from build123d import *

# Parameters (mm, degrees)
SKETCH1_W           = 13
SKETCH1_H           = 16.2
BOSS_EXTRUDE1_DEPTH = 12.5
SKETCH2_W           = 2
SKETCH2_H           = 16.2
BOSS_EXTRUDE5_DEPTH = 6.5
SKETCH7_R           = 2.9
BOSS_EXTRUDE6_DEPTH = 2.5
SKETCH8_R           = 1.9
BOSS_EXTRUDE7_DEPTH = 8
SKETCH9_W           = 5
SKETCH9_H           = 16.2
BOSS_EXTRUDE8_DEPTH = 4
SKETCH10_W          = 0.8
SKETCH10_H          = 9.3
CUT_EXTRUDE3_DEPTH  = 6
SKETCH11_R          = 0.75
BOSS_EXTRUDE9_DEPTH = 2.5


with BuildPart() as part:
    # Sketch1 → Boss-Extrude1 (new body)
    with BuildSketch(Plane.XY):
        Rectangle(SKETCH1_W, SKETCH1_H)
    extrude(amount=-BOSS_EXTRUDE1_DEPTH)

    # Sketch2 → Boss-Extrude5 (add)
    with BuildSketch(Plane(origin=(0, 0, -12.5), x_dir=(-1, 0, 0), z_dir=(0, 0, -1))):
        with Locations((-7.5, 0)):
            Rectangle(SKETCH2_W, SKETCH2_H)
        with Locations((7.5, 0)):
            Rectangle(SKETCH2_W, SKETCH2_H)
    extrude(amount=-BOSS_EXTRUDE5_DEPTH)

    # Sketch7 → Boss-Extrude6 (add)
    with BuildSketch(Plane.XZ.offset(8.1)):
        with Locations(Location((2, -3, 0), (0, 0, 270))):
            Circle(SKETCH7_R)
    extrude(amount=BOSS_EXTRUDE6_DEPTH)

    # Sketch8 → Boss-Extrude7 (add)
    with BuildSketch(Plane.XZ.offset(10.6)):
        with Locations(Location((2, -3, 0), (0, 0, 270))):
            Circle(SKETCH8_R)
    extrude(amount=BOSS_EXTRUDE7_DEPTH)

    # Sketch9 → Boss-Extrude8 (add)
    with BuildSketch(Plane(origin=(0, 0, -12.5), x_dir=(-1, 0, 0), z_dir=(0, 0, -1))):
        with Locations((-11, 0)):
            Rectangle(SKETCH9_W, SKETCH9_H)
        with Locations((11, 0)):
            Rectangle(SKETCH9_W, SKETCH9_H)
    extrude(amount=-BOSS_EXTRUDE8_DEPTH)

    # Sketch10 → Cut-Extrude3 (cut)
    with BuildSketch(Plane.XY):
        with Locations((6.1, 3.45)):
            Rectangle(SKETCH10_W, SKETCH10_H)
        with Locations((-6.1, 3.45)):
            Rectangle(SKETCH10_W, SKETCH10_H)
    extrude(amount=-CUT_EXTRUDE3_DEPTH, mode=Mode.SUBTRACT)

    # Sketch11 → Boss-Extrude9 (add)
    with BuildSketch(Plane.XY.offset(-8.5)):
        with Locations((-10.9, -3.1)):
            Circle(SKETCH11_R)
        with Locations(Location((10.9, -3.1, 0), (0, 0, 180))):
            Circle(SKETCH11_R)
    extrude(amount=BOSS_EXTRUDE9_DEPTH)


solid = part.part
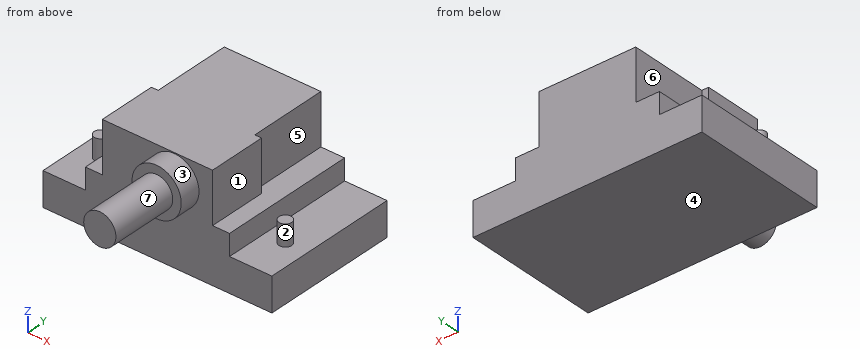
Read the model definition and answer for the solid it produces. Units are mm, in the model's axes. Face numbers are marked on the shaded views. A direction names the side the tool comes from. Give positions to 0.01 mm unless a question says otherwise; leave off trailing zeros. Loops run counter-clockwise (first coordinate to the right, second up) from the corner with the lowest first, then second, coordinate; pieces in that order, holes last. Notation, with made-up numbers: (22.5, -21) -> (80.5, -21) arc R18 cw to (80.5, -7) -> close; hole circle Ø9 at (2, 17.25). An arc over 180 degrees is marked (long way). Use a Markdown table: item, result.
Q1. Section A-A, the plane x = 2 is taken. Determine the outline of the cut face in (y, z), then the cut area to 3 significant figures.
Solved:
| item | result |
|---|---|
| outline | (-18.6, -4.9) -> (-10.6, -4.9) -> (-10.6, -5.9) -> (-8.1, -5.9) -> (-8.1, -12.5) -> (8.1, -12.5) -> (8.1, 0) -> (-8.1, 0) -> (-8.1, -0.1) -> (-10.6, -0.1) -> (-10.6, -1.1) -> (-18.6, -1.1) -> close |
| area | 247 mm^2 |
Q2. Section B-B, the plane y = -5 is taken. Determine the outline of the cut face in (x, z), then the cut area to 4 significant figures.
Solved:
| item | result |
|---|---|
| outline | (-13.5, -12.5) -> (13.5, -12.5) -> (13.5, -8.5) -> (8.5, -8.5) -> (8.5, -6) -> (6.5, -6) -> (6.5, 0) -> (-6.5, 0) -> (-6.5, -6) -> (-8.5, -6) -> (-8.5, -8.5) -> (-13.5, -8.5) -> close |
| area | 228.5 mm^2 |
Q3. Each of these flat-tipped pins is pushed along its axis until it touches: pin 1 (0.8 mm diameter, centred on y = 3.5, z = -6.5, fed in from -X); pin 2 (1.4 mm diameter, centred on x = 7.5, y = 2.5, fed in from +Z); pin 3 (1.8 mm diameter, centred on y = 2.5, z = -3.5, fed in from +X); pin 4 (0.9 mm diameter, centred on x = -6, z = -4, fed in from +Y). Where does it stop, or does it pass through?
Solved:
| item | result |
|---|---|
| pin 1 | stops at x = -8.5 |
| pin 2 | stops at z = -6 |
| pin 3 | stops at x = 5.7 |
| pin 4 | stops at y = 8.1 |
Q4. Find the intervals of material crossed by line 1 along X through (y, z) = (-1, -5.25); line 2 along Y through (x, z) = (5.5, -9.75); line 3 along X through (y, z) = (-8, -1.5), in increasing order.
Solved:
| item | result |
|---|---|
| line 1 | x = -5.7 to 5.7 |
| line 2 | y = -8.1 to 8.1 |
| line 3 | x = -6.5 to 6.5 |
Q5. A tool of negligible diameter and unlimited length cuts with its end or side. For the marked faces 4, 5, 6 and 7, from which of +Z, -Z, +X, -X, +Y, -Y can it reach the whole face along a straight path? Write none if from no direction.
Solved:
| item | result |
|---|---|
| face 4 | -Z, +X, -X, +Y, -Y |
| face 5 | +Z, +X, +Y |
| face 6 | +Z, -X, +Y |
| face 7 | -Y |
Q6. Section C-C, the plane z = -3 is taken. Determine the outline of the cut face in (x, y), then the cut area to 3 significant figures.
Solved:
| item | result |
|---|---|
| outline | (-6.5, -8.1) -> (-0.9, -8.1) -> (-0.9, -10.6) -> (0.1, -10.6) -> (0.1, -18.6) -> (3.9, -18.6) -> (3.9, -10.6) -> (4.9, -10.6) -> (4.9, -8.1) -> (6.5, -8.1) -> (6.5, -1.2) -> (5.7, -1.2) -> (5.7, 8.1) -> (-5.7, 8.1) -> (-5.7, -1.2) -> (-6.5, -1.2) -> close |
| area | 241 mm^2 |
Q7. Section D-D, the plane x = -10.9 is taken. Determine the outline of the cut face in (y, z).
Solved:
| item | result |
|---|---|
| outline | (-8.1, -12.5) -> (8.1, -12.5) -> (8.1, -8.5) -> (-2.35, -8.5) -> (-2.35, -6) -> (-3.85, -6) -> (-3.85, -8.5) -> (-8.1, -8.5) -> close |
Q8. Determine the mould class of the marked faces 1, 2 and 3 for opening direction X: pulls with the +X half, pulls with the -X half, needs draft (parallel to the pull), parting line crosses it, or undercut.
Solved:
| item | result |
|---|---|
| face 1 | pulls with the +X half |
| face 2 | undercut |
| face 3 | parting line crosses it |
